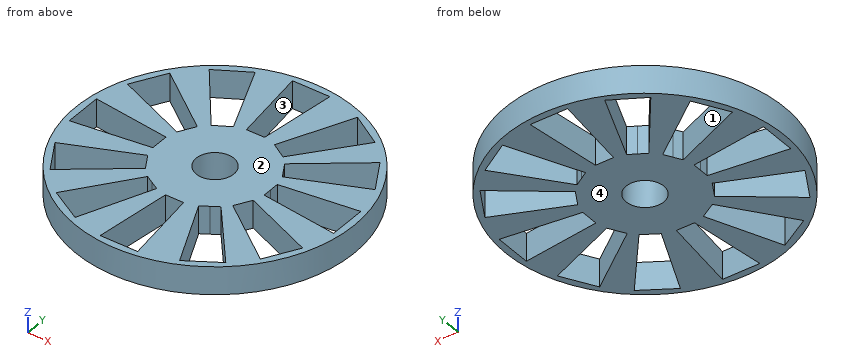
```python
from build123d import *

# Parameters (mm, degrees)
ESBO_O1_R                = 10
ESBO_O1_R_2              = 1.35
RESSALTO_EXTRUS_O2_DEPTH = 2


with BuildPart() as part:
    # Esboço1 → Ressalto-extrusão2 (new body)
    with BuildSketch(Plane.XY):
        Circle(ESBO_O1_R)
        Circle(ESBO_O1_R_2, mode=Mode.SUBTRACT)
        Polygon((-1.345467814, 9.5), (1.345467814, 9.5), (0.65, 4), (0, 4), (-0.65, 4), align=None, mode=Mode.SUBTRACT)
        Polygon((2.655029784, 3.061587308), (6.136998996, 7.375467915), (3.847574626, 8.789565014), (1.549001215, 3.744742346), (2.102015499, 3.403164827), align=None, mode=Mode.SUBTRACT)
        Polygon((-1.436650808, 3.789265688), (-3.5837744, 8.900384525), (-5.914346634, 7.555182826), (-2.562558048, 3.139394249), (-1.999604428, 3.464329969), align=None, mode=Mode.SUBTRACT)
        Polygon((-3.463644773, 2.000791065), (-3.788773321, 1.43794879), (-8.899156331, 3.58682314), (-7.553156341, 5.91693442), (-3.138516225, 2.563633341), align=None, mode=Mode.SUBTRACT)
        Polygon((-3.999999765, 0.001370256), (-4.000222432, -0.648629706), (-9.500460351, -1.342213377), (-9.499538534, 1.348722092), (-3.999777099, 0.651370218), align=None, mode=Mode.SUBTRACT)
        Polygon((-3.465014758, -1.998417556), (-3.140271905, -2.561482454), (-7.557208424, -5.911758154), (-8.901611674, -3.580725239), (-3.789757611, -1.435352658), align=None, mode=Mode.SUBTRACT)
        Polygon((-1.999604428, -3.464329969), (-1.436650808, -3.789265688), (-3.5837744, -8.900384525), (-5.914346634, -7.555182826), (-2.562558048, -3.139394249), align=None, mode=Mode.SUBTRACT)
        Polygon((-0.65, -4), (-1.345467814, -9.5), (1.345467814, -9.5), (0.65, -4), (0, -4), align=None, mode=Mode.SUBTRACT)
        Polygon((2.102015499, -3.403164827), (2.655029784, -3.061587308), (6.136998996, -7.375467915), (3.847574626, -8.789565014), (1.549001215, -3.744742346), align=None, mode=Mode.SUBTRACT)
        Polygon((3.465014758, -1.998417556), (3.789757611, -1.435352658), (8.901611674, -3.580725239), (7.557208424, -5.911758154), (3.140271905, -2.561482454), align=None, mode=Mode.SUBTRACT)
        Polygon((3.999999765, 0.001370256), (3.999777099, 0.651370218), (9.499538534, 1.348722092), (9.500460351, -1.342213377), (4.000222432, -0.648629706), align=None, mode=Mode.SUBTRACT)
        Polygon((3.463644773, 2.000791065), (3.138516225, 2.563633341), (7.553156341, 5.91693442), (8.899156331, 3.58682314), (3.788773321, 1.43794879), align=None, mode=Mode.SUBTRACT)
    extrude(amount=RESSALTO_EXTRUS_O2_DEPTH)


solid = part.part
```
Can you work these out from the model? Positions are in its coordinate system, mm. Face numbers are marked on the shaded views. A direction names the side the tool comes from. Coordinates: 2 decimals unless noted, no trailing zeros. Write each loop counter-clockwise with the first axis right and the second up, starting at its lowest first coordinate (ties: lowest second). Pieces come first, ordered by that corner, then holes. Notation, with made-up numbers: M 14,72.25 L 48,72.25 A8 ccw 48,83.25 Z; hole C -13,-18 d1. An arc over 180 degrees is marked long. Answer as CSV lines item,"result".
Item 1: I'm going to push flat-ended pins straight in: P1, Ø1.6, axis at x = 0, y = 0, coming from the -Z side; P2, Ø1, axis at y = 6, z = 0.5, coming from the -X side. Where does each tip first touch, or does it pass through?
Geometry results:
P1,"passes through"
P2,"stops at x = -8.35"
Item 2: On a 3-axis mill with a long thin cutter (end or side, diameter ignored), from which of +Z, -Z, +X, -X, +Y, -Y can I reach the whole of each face in a straight line? I mean the marked faces 1 and 2. Say none if no direction works.
Geometry results:
face 1,"+Z, -Z"
face 2,"+Z, +X, -X, +Y, -Y"
Item 3: Imagine slicing it at B-B on x = 5.25. List the corners of the cut face in (y, z) for me, plus the area to 3 significant figures.
Geometry results:
outline,"M -8.51,0 L -7.92,0 L -7.92,2 L -8.51,2 Z; M -6.28,0 L -4.16,0 L -4.16,2 L -6.28,2 Z; M -2.05,0 L -0.81,0 L -0.81,2 L -2.05,2 Z; M 0.81,0 L 2.05,0 L 2.05,2 L 0.81,2 Z; M 4.17,0 L 6.28,0 L 6.28,2 L 4.17,2 Z; M 7.92,0 L 8.51,0 L 8.51,2 L 7.92,2 Z"
area,"15.8 mm2"
Item 4: Imagine slicing it at C-C on z = 1.2. State how many separate pieces and enclosed holes the cut face has, plus the area to 3 significant figures.
Geometry results:
separate pieces,"1"
enclosed holes,"13"
area,"177 mm2"
Item 5: We'd pull the mould along X, two halves only. Please class the marked faces 3 and 4: +X half, -X half, draft (parallel to the pull), parting line (faces both ways), or undercut.
Geometry results:
face 3,"undercut"
face 4,"draft"
Item 6: Please list where these lines run through material, in increasing order: line 1 along Y through (x, z) = (0, 1.45); line 2 along X through (y, z) = (4.25, 1.8); line 3 along Y through (x, z) = (4.5, 0.7).
Geometry results:
line 1,"y = -10 to -9.5, -4 to -1.35, 1.35 to 4, 9.5 to 10"
line 2,"x = -9.05 to -8.52, -5.36 to -3.41, -1.63 to -0.68, 0.68 to 1.78, 3.61 to 5.36, 8.52 to 9.05"
line 3,"y = -8.93 to -8.39, -5.35 to -3.59, -1.73 to -0.71, 0.71 to 1.74, 3.6 to 5.35, 8.39 to 8.93"
Item 7: Imagine slicing it at A-A on x = 0. List the corners of the cut face in (y, z) for me.
Geometry results:
outline,"M -10,0 L -9.5,0 L -9.5,2 L -10,2 Z; M -4,0 L -1.35,0 L -1.35,2 L -4,2 Z; M 1.35,0 L 4,0 L 4,2 L 1.35,2 Z; M 9.5,0 L 10,0 L 10,2 L 9.5,2 Z"
